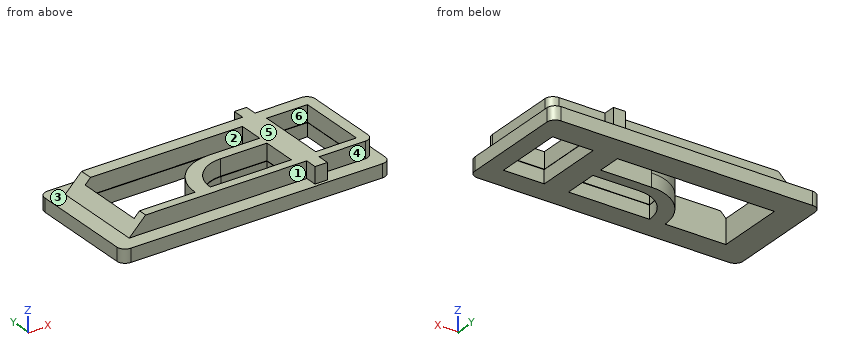
from build123d import *

# Parameters (mm, degrees)
SKETCH1_W           = 32.68
SKETCH1_H           = 14.5
BOSS_EXTRUDE2_DEPTH = 1.62
SKETCH3_W           = 4.962331447
SKETCH3_H           = 8.5
SKETCH3_W_2         = 1.5
SKETCH3_H_2         = 1.444155173
SKETCH3_H_3         = 1.444155172
BOSS_EXTRUDE3_DEPTH = 2
CUT_EXTRUDE1_START  = -2
SKETCH4_W           = 4.962331446
SKETCH4_H           = 8.5
CUT_EXTRUDE1_DEPTH  = 2
FILLET1_R           = 1
CHAMFER1_SIZE       = 2.3


with BuildPart() as part:
    # Sketch1 → Boss-Extrude2 (new body)
    with BuildSketch(Plane.XY):
        Rectangle(SKETCH1_W, SKETCH1_H)
    extrude(amount=-BOSS_EXTRUDE2_DEPTH)

    # Sketch3 → Boss-Extrude3 (add)
    # profile 1 of 3: a face of its own
    with BuildSketch(Plane.XY):
        Polygon((7.357218521, 5.676374473), (-14.565223124, 5.676374473), (-14.565223124, -5.435315182), (7.357218521, -5.435315182), (8.857218521, -5.435315182), (15.486501014, -5.435315182), (15.486501014, 5.676374473), (8.857218521, 5.676374473), align=None)
        with BuildLine():
            Line((6.231943334, 4.121127688), (6.231943334, 2.506027416))
            Line((6.231943334, 2.506027416), (6.231943334, 1.135297756))
            Line((6.231943334, 1.135297756), (0.017218521, 1.135297756))
            ThreePointArc((0.017218521, 1.135297756), (-3.881888527, -0.479765264), (-5.496951548, -4.378872312))
            Line((-5.496951548, -4.378872312), (-12.923950607, -4.378872312))
            Line((-12.923950607, -4.378872312), (-12.923950607, 4.121127688))
            Line((-12.923950607, 4.121127688), (6.231943334, 4.121127688))
        make_face(mode=Mode.SUBTRACT)
        with BuildLine():
            Line((6.231943334, -0.128872312), (6.231943334, -4.378872312))
            Line((6.231943334, -4.378872312), (-3.642781479, -4.378872312))
            ThreePointArc((-3.642781479, -4.378872312), (-2.397985299, -1.373668492), (0.607218521, -0.128872312))
            Line((0.607218521, -0.128872312), (6.231943334, -0.128872312))
        make_face(mode=Mode.SUBTRACT)
        with Locations((11.670056084, -0.128872312)):
            Rectangle(SKETCH3_W, SKETCH3_H, mode=Mode.SUBTRACT)
    # profile 2 of 3: a face of its own
    with BuildSketch(Plane.XY):
        with Locations((8.107218521, -6.157392769)):
            Rectangle(SKETCH3_W_2, SKETCH3_H_2)
    # profile 3 of 3: a face of its own
    with BuildSketch(Plane.XY):
        with Locations((8.107218521, 6.398452059)):
            Rectangle(SKETCH3_W_2, SKETCH3_H_3)
    extrude(amount=BOSS_EXTRUDE3_DEPTH)

    # Sketch4 → Cut-Extrude1 (cut)
    with BuildSketch(Plane.XY.offset(CUT_EXTRUDE1_START)):
        with BuildLine():
            Line((6.197506292, 1.135297756), (6.197506292, 2.437153333))
            Line((6.197506292, 2.437153333), (6.197506292, 4.052253605))
            Line((6.197506292, 4.052253605), (-12.923950607, 4.052253605))
            Line((-12.923950607, 4.052253605), (-12.923950607, -4.378872312))
            Line((-12.923950607, -4.378872312), (-5.530958441, -4.378872312))
            ThreePointArc((-5.530958441, -4.378872312), (-5.371289583, -3.128657844), (-4.931903418, -1.947357645))
            ThreePointArc((-4.931903418, -1.947357645), (-2.898110461, 0.301611474), (0.017218521, 1.135297756))
            Line((0.017218521, 1.135297756), (6.197506292, 1.135297756))
        make_face()
        with BuildLine():
            ThreePointArc((-3.677218521, -4.447746395), (-2.432422341, -1.442542575), (0.572781479, -0.197746395))
            Line((0.572781479, -0.197746395), (6.197506292, -0.197746395))
            Line((6.197506292, -0.197746395), (6.197506292, -4.447746395))
            Line((6.197506292, -4.447746395), (-3.677218521, -4.447746395))
        make_face()
        with Locations((11.635619042, -0.197746395)):
            Rectangle(SKETCH4_W, SKETCH4_H)
    extrude(amount=CUT_EXTRUDE1_DEPTH, mode=Mode.SUBTRACT)

    # Fillet1
    fillet1_edges = [part.edges().sort_by_distance(p)[0] for p in [
        (15.486501014, -5.435315182, 1),
        (15.486501014, 5.676374473, 1),
        (16.34, -7.25, -0.81),
        (-16.34, -7.25, -0.81),
        (-16.34, 7.25, -0.81),
        (16.34, 7.25, -0.81),
    ]]
    fillet(fillet1_edges, radius=FILLET1_R)

    # Chamfer1
    # the kernel refuses this chamfer: 2.3 mm, written as the material it takes off along each edge
    with BuildSketch(Plane(origin=(-14.565223124, 11.591245345, 2), x_dir=(-0.02749587661058623, 0, -0.9996219169112968), z_dir=(0, -1, 0))) as chamfer1_piece_1_section:
        Polygon((CHAMFER1_SIZE * 0.999621916911, CHAMFER1_SIZE * 0.0274958766106), (-CHAMFER1_SIZE * 0.0274958766106, CHAMFER1_SIZE * 0.999621916911), (0, 0), align=None)
    chamfer1_piece_1 = extrude(amount=22.9414314, mode=Mode.PRIVATE)
    chamfer1_piece_1 = split(chamfer1_piece_1, bisect_by=Plane(origin=(-13.786723821, 0.120529645, 0), z_dir=(0, 0, 1)), keep=Keep.TOP, mode=Mode.PRIVATE)
    add(chamfer1_piece_1, mode=Mode.SUBTRACT)


solid = part.part
Geometry check sheet. Reference: the model listing, model coordinates, mm. Face numbers are marked on the shaded views. A direction names the side the tool comes from. Round coordinates to 2 decimals unless told otherwise and drop trailing zeros. Loops run counter-clockwise (first coordinate to the right, second up) from the corner with the lowest first, then second, coordinate; pieces in that order, holes last.
Item 1: Cross-section at C-C on z = -0.85. Record the boundary of the cut face in (x, y), then the cut area to 3 significant figures.
Item 2: Access from +Z, -Z, +X, -X, +Y, -Y to the whole of each face (thin tool, end or side, straight path). Record for the marked faces 4, 5 and 6.
Item 3: Gauge pin test, flat ends, axial feed: pin 1 (2 mm diameter, centred on x = 2.5, y = -3.5, fed in from +Z); pin 2 (2.5 mm diameter, centred on x = 11, y = 1, fed in from +Z); pin 3 (1 mm diameter, centred on x = -5.5, z = 1, fed in from +Y); pin 4 (0.6 mm diameter, centred on x = 10.5, z = 1, fed in from -Y). Record the tip position at first contact, or that the pin passes through.
Item 4: Cross-section at A-A on x = 9.5. Record the boundary of the cut face in (y, z).
Item 5: Cross-section at D-D on y = -5.75. Record the boundary of the cut face in (x, z).
Item 6: Thickness scan on line 1 (Y direction, x = 5, z = -1.05); line 2 (Y direction, x = -12.5, z = -0.5); line 3 (X direction, y = 3.5, z = -0.4). Record the ranges inside material, lowest first.
Item 7: Cross-section at B-B on y = 1.75. Count the separate pieces of the cut face and the enclosed holes in it, then the cut area to 3 significant figures.
Item 8: Mould release check, pull along Y, two halves, no side actions. Record for the marked faces 1, 2 and 3: pulls with the +Y half, pulls with the -Y half, needs draft (parallel to the pull), parting line crosses it, or undercut.
Answer sheet:
1. outline: (-16.34, -6.25) arc R1 ccw to (-15.34, -7.25) - (15.34, -7.25) arc R1 ccw to (16.34, -6.25) - (16.34, 6.25) arc R1 ccw to (15.34, 7.25) - (-15.34, 7.25) arc R1 ccw to (-16.34, 6.25) - close; hole (-12.92, -4.38) - (-5.53, -4.38) arc R5.51 cw to (-4.93, -1.95) arc R5.51 cw to (0.02, 1.14) - (6.2, 1.14) - (6.2, 4.05) - (-12.92, 4.05) - close; hole (-3.68, -4.45) - (6.2, -4.45) - (6.2, -0.2) - (0.57, -0.2) arc R4.25 ccw to start; hole (9.15, -4.45) - (14.12, -4.45) - (14.12, 4.05) - (9.15, 4.05) - close
1. area: 290 mm2
2. face 4: +Z, +X, -Y
2. face 5: +Z, +X, -X, +Y, -Y
2. face 6: +Z
3. pin 1: stops at z = 2
3. pin 2: passes through
3. pin 3: stops at y = 5.68
3. pin 4: stops at y = -5.44
4. outline: (-7.25, -1.62) - (-4.45, -1.62) - (-4.45, 0) - (-4.38, 0) - (-4.38, 2) - (-5.44, 2) - (-5.44, 0) - (-7.25, 0) - close; (4.05, -1.62) - (7.25, -1.62) - (7.25, 0) - (5.68, 0) - (5.68, 2) - (4.12, 2) - (4.12, 0) - (4.05, 0) - close
5. outline: (-16.34, -1.62) - (16.34, -1.62) - (16.34, 0) - (8.86, 0) - (8.86, 2) - (7.36, 2) - (7.36, 0) - (-16.34, 0) - close
6. line 1: y = -7.25 to -4.45, -0.2 to 1.14, 4.05 to 7.25
6. line 2: y = -7.25 to -4.38, 4.05 to 7.25
6. line 3: x = -16.34 to -12.92, 6.2 to 9.15, 14.12 to 16.34
7. separate pieces: 3
7. enclosed holes: 0
7. area: 23.4 mm2
8. face 1: pulls with the -Y half
8. face 2: undercut
8. face 3: needs draft
